```python
from build123d import *

# Parameters (mm, degrees)
BOSS_EXTRUDE1_DEPTH = 38
CUT_EXTRUDE1_DEPTH  = 4
CUT_EXTRUDE2_DEPTH  = 4


with BuildPart() as part:
    # Sketch1 → Boss-Extrude1 (new body)
    with BuildSketch(Plane(origin=(0, 0, 0), x_dir=(0, 0, -1), z_dir=(1, 0, 0))):
        Polygon((0, 20), (0, 0), (20, 0), (20, 3), (3, 3), (3, 20), align=None)
    extrude(amount=-BOSS_EXTRUDE1_DEPTH)

    # Sketch2 → Cut-Extrude1 (cut, through all)
    with BuildSketch(Plane(origin=(0, 0, -3), x_dir=(-1, 0, 0), z_dir=(0, 0, -1))):
        with BuildLine():
            Line((4.75, 12.75), (9.75, 12.75))
            ThreePointArc((9.75, 12.75), (12.5, 10), (9.75, 7.25))
            Line((9.75, 7.25), (4.75, 7.25))
            ThreePointArc((4.75, 7.25), (2, 10), (4.75, 12.75))
        make_face()
    cut_extrude1 = extrude(amount=-CUT_EXTRUDE1_DEPTH, mode=Mode.SUBTRACT)

    # Sketch3 → Cut-Extrude2 (cut, through all)
    with BuildSketch(Plane(origin=(0, 3, 0), x_dir=(1, 0, 0), z_dir=(0, 1, 0))):
        with BuildLine():
            Line((-4.75, 12.25), (-9.75, 12.25))
            ThreePointArc((-9.75, 12.25), (-12.5, 15), (-9.75, 17.75))
            Line((-9.75, 17.75), (-4.75, 17.75))
            ThreePointArc((-4.75, 17.75), (-2, 15), (-4.75, 12.25))
        make_face()
    cut_extrude2 = extrude(amount=-CUT_EXTRUDE2_DEPTH, mode=Mode.SUBTRACT)

    # Mirror1: Cut-Extrude1 across plane
    add(cut_extrude1.mirror(Plane(origin=(-19, 0, 0), x_dir=(0, 0, 1), z_dir=(1, 0, 0))), mode=Mode.SUBTRACT)

    # Mirror2: Cut-Extrude2 across plane
    add(cut_extrude2.mirror(Plane(origin=(-19, 0, 0), x_dir=(0, 0, 1), z_dir=(1, 0, 0))), mode=Mode.SUBTRACT)


solid = part.part
```
Check sheet for the modelled part. Datum: model origin and axes. Units: mm. A direction names the side the tool comes from. Coordinates: 2 decimals unless noted, no trailing zeros. Loops run counter-clockwise (first coordinate to the right, second up) from the corner with the lowest first, then second, coordinate; pieces in that order, holes last.
1) Sectioned sample at D-D (x = -34). Record the boundary of the cut face in (y, z).
2) Material ranges on probe 1 along Y at (x, z) = (-28.5, -8); probe 2 along Z at (x, y) = (-22, 15); probe 3 along Y at (x, z) = (-27.5, -1.25), recorded low to high.
3) Release check for a two-part mould opening along Z. For faces 1 (the face through (-36, 10, -2)), 2 (the face through (-25.5, 1.5, -14.9)), 3 (the face through (-19, 11, -3)), 4 (the face through (-31, 2, -17.75)) record: released by +Z, released by -Z, zero draft, split by the parting line, or undercut.
4) Sectioned sample at C-C (x = -14.5). Record the boundary of the cut face in (y, z).
5) Sectioned sample at A-A (y = 10). Record the boundary of the cut face in (x, z).
6) Gauge pin test, flat ends, axial feed: pin 1 (1 mm diameter, centred on x = -25.5, y = 4, fed in from -Z); pin 2 (3 mm diameter, centred on x = -7, z = -15, fed in from -Y); pin 3 (3.5 mm diameter, centred on x = -31.5, y = 1, fed in from +Z); pin 4 (6 mm diameter, centred on x = -24.5, z = -7.5, fed in from +Y). Record the tip position at first contact, or that the pin passes through.
7) Access from +Z, -Z, +X, -X, +Y, -Y to the whole of each face (thin tool, end or side, straight path). Record for faces 5 (the face through (-19, 20, -2)), 6 (the face through (-31, 7.25, -2)), 7 (the face through (-31, 2, -12.25)).
8) Sectioned sample at B-B (z = -15). Record the boundary of the cut face in (x, y), and give its area (3 significant figures).
Check sheet entries:
1. outline: (0, -20) - (3, -20) - (3, -17.65) - (0, -17.65) - close; (0, -12.35) - (3, -12.35) - (3, -3) - (7.35, -3) - (7.35, 0) - (0, 0) - close; (12.65, -3) - (20, -3) - (20, 0) - (12.65, 0) - close
2. probe 1: y = 0 to 3
2. probe 2: z = -3 to 0
2. probe 3: y = 0 to 7.35, 12.65 to 20
3. face 1: zero draft
3. face 2: undercut
3. face 3: released by -Z
3. face 4: undercut
4. outline: (0, -20) - (3, -20) - (3, -3) - (20, -3) - (20, 0) - (0, 0) - close
5. outline: (-38, -3) - (-36, -3) - (-36, 0) - (-38, 0) - close; (-25.5, -3) - (-12.5, -3) - (-12.5, 0) - (-25.5, 0) - close; (-2, -3) - (0, -3) - (0, 0) - (-2, 0) - close
6. pin 1: stops at z = -3
6. pin 2: passes through
6. pin 3: stops at z = 0
6. pin 4: stops at y = 3
7. face 5: +Z, -Z, +X, -X, +Y
7. face 6: +Z, -Z
7. face 7: +Y, -Y
8. outline: (-38, 0) - (-36, 0) - (-36, 3) - (-38, 3) - close; (-25.5, 0) - (-12.5, 0) - (-12.5, 3) - (-25.5, 3) - close; (-2, 0) - (0, 0) - (0, 3) - (-2, 3) - close
8. area: 51.0 mm2
